Autodesk Inventor part; units mm, degrees
ref_plane "YZ Plane" through (0, 0, 0) normal (1, 0, 0) x (0, 1, 0)
ref_plane "XZ Plane" through (0, 0, 0) normal (0, 1, 0) x (-1, 0, 0)
ref_plane "XY Plane" through (0, 0, 0) normal (0, 0, 1) x (1, 0, 0)
sketch "Sketch1" plane through (0, 0, 0) normal (0, 1, 0) x (-1, 0, 0)
  circle A0 centre (0, 0) radius 12.7
  dimension "d0" = 25.4
extrude "Extrusion1" add sketch "Sketch1" along normal blind 25.4
sketch "Sketch2" plane through (0, 25.4, 0) normal (0, 1, 0) x (1, 0, 0)
  circle A0 centre (0, 0) radius 2.4685
hole "Hole1" at (0, 25.4, 0) direction (0, -1, 0) diameter 8.4328 depth 19.05 tip angle 118
sketch "Sketch3" plane through (0, 0, 0) normal (0, -1, 0) x (1, 0, 0)
  circle A0 centre (0, 0) radius 4.2164
  circle A1 centre (0, 0) radius 3.0691
hole "Hole2" at (0, 0, 0) direction (0, 1, 0) diameter 6.4008 depth 12.7 tip angle 118
properties part number "spacer"
The listing builds one solid part. Answer for the finished solid, in the listing's coordinates (mm). Coordinates: 2 decimals unless noted, no trailing zeros. Loops run counter-clockwise (first coordinate to the right, second up) from the corner with the lowest first, then second, coordinate; pieces in that order, holes last. Notation, with made-up numbers: (58, 11) -> (114, 11) arc R30 ccw to (114, 41) -> close; hole circle Ø4 at (9.25, 81.25). An arc over 180 degrees is marked (long way). Return JSON: item names as keys, results as strings. Group by question number.
(1) A cutting plane is placed at A-A on x = 0. Write down the section's boundary in (y, z).
(2) Determine the mould class of faces 1 (the cylindrical face through (2.75, 12.52, 12.4)), 2 (the cylindrical face through (1.95, 2.91, 2.54)), 3 (the flat face through (-5, 25.4, 0)), 4 (the cylindrical face through (-4.18, 15.74, -0.55)) for opening direction Z: released by +Z, released by -Z, zero draft, split by the parting line, or undercut.
(3) A cutting plane is placed at C-C on y = 19. Write down the section's boundary in (x, z).
(4) A cutting plane is placed at B-B on z = 0. Write down the section's boundary in (x, y).
(5) Given pin 1 Ø6 at (x, z) = (0, 0) entering from -Y; pin 2 Ø2 at (y, z) = (8, -8.5) entering from -X; pin 3 Ø2 at (x, y) = (-9.5, 6.5) entering from -Z; pin 4 Ø1 at (x, y) = (-8.5, 14.5) entering from -Z, each flat-ended and moving along its own axis, determine where each tip first touches the part or whether it passes through.
(6) A cutting plane is placed at D-D on x = 10.75. Write down the section's boundary in (y, z), and give its area (3 significant figures).
(7) Find the intervals of material crossed by probe 1 along Z at (x, y) = (0, 4.05); probe 2 along X at (y, z) = (12.75, -3.25); probe 3 along Z at (x, y) = (2.5, 7.5), in increasing order. Write a range as from..to.
The answers:
{
 "1": {"outline": "(0, -12.7) -> (25.4, -12.7) -> (25.4, -4.22) -> (6.35, -4.22) -> (5.74, -3.2) -> (0, -3.2) -> close; (0, 3.2) -> (5.74, 3.2) -> (6.35, 4.22) -> (25.4, 4.22) -> (25.4, 12.7) -> (0, 12.7) -> close"},
 "2": {"face 1": "split by the parting line", "face 2": "undercut", "face 3": "zero draft", "face 4": "undercut"},
 "3": {"outline": "circle Ø25.4 at (0, 0); hole circle Ø8.43 at (0, 0)"},
 "4": {"outline": "(-12.7, 0) -> (-3.2, 0) -> (-3.2, 5.74) -> (-4.22, 6.35) -> (-4.22, 25.4) -> (-12.7, 25.4) -> close; (3.2, 0) -> (12.7, 0) -> (12.7, 25.4) -> (4.22, 25.4) -> (4.22, 6.35) -> (3.2, 5.74) -> close"},
 "5": {"pin 1": "passes through", "pin 2": "stops at x = -10.25", "pin 3": "stops at z = -9.44", "pin 4": "stops at z = -9.86"},
 "6": {"outline": "(0, -6.76) -> (25.4, -6.76) -> (25.4, 6.76) -> (0, 6.76) -> close", "area": "344 mm^2"},
 "7": {"probe 1": "z = -12.7..-3.2, 3.2..12.7", "probe 2": "x = -12.28..-2.69, 2.69..12.28", "probe 3": "z = -12.45..-3.4, 3.4..12.45"}
}
